```python
from build123d import *

# Parameters (mm, degrees)
F_01_RAIL_BASE_PROFILE_W   = 340
F_01_RAIL_BASE_PROFILE_H   = 130
F_01_RAIL_BASE_PROFILE_R   = 4.5
F_01_RAIL_BASE_PROFILE_W_2 = 281
F_01_RAIL_BASE_PROFILE_H_2 = 62
F_01_RAIL_BASE_DEPTH       = 10
F_02_GUIDE_RAIL_PROFILES_W = 326.4
F_02_GUIDE_RAIL_PROFILES_H = 10
F_02_GUIDE_RAILS_DEPTH     = 42


with BuildPart() as part:
    # 01_Rail_Base_Profile → 01_Rail_Base (new body)
    with BuildSketch(Plane(origin=(0, 0, 0), x_dir=(1, 0, 0), z_dir=(0, 1, 0))):
        Rectangle(F_01_RAIL_BASE_PROFILE_W, F_01_RAIL_BASE_PROFILE_H)
        with Locations(Location((-145, -52, 0), (0, 0, 270))):
            Circle(F_01_RAIL_BASE_PROFILE_R, mode=Mode.SUBTRACT)
        with Locations(Location((-145, 52, 0), (0, 0, 270))):
            Circle(F_01_RAIL_BASE_PROFILE_R, mode=Mode.SUBTRACT)
        with Locations(Location((145, -52, 0), (0, 0, 270))):
            Circle(F_01_RAIL_BASE_PROFILE_R, mode=Mode.SUBTRACT)
        with Locations(Location((145, 52, 0), (0, 0, 270))):
            Circle(F_01_RAIL_BASE_PROFILE_R, mode=Mode.SUBTRACT)
        Rectangle(F_01_RAIL_BASE_PROFILE_W_2, F_01_RAIL_BASE_PROFILE_H_2, mode=Mode.SUBTRACT)
    extrude(amount=F_01_RAIL_BASE_DEPTH)

    # 02_Guide_Rail_Profiles → 02_Guide_Rails (add)
    with BuildSketch(Plane(origin=(0, 0, 0), x_dir=(1, 0, 0), z_dir=(0, 1, 0))):
        with Locations((0, 52)):
            Rectangle(F_02_GUIDE_RAIL_PROFILES_W, F_02_GUIDE_RAIL_PROFILES_H)
        with Locations((0, -52)):
            Rectangle(F_02_GUIDE_RAIL_PROFILES_W, F_02_GUIDE_RAIL_PROFILES_H)
    extrude(amount=F_02_GUIDE_RAILS_DEPTH)


solid = part.part
```
Verification items for the finished model (mm, model axes). A direction names the side the tool comes from. Coordinates: 2 decimals unless noted, no trailing zeros. Write each loop counter-clockwise with the first axis right and the second up, starting at its lowest first coordinate (ties: lowest second). Pieces come first, ordered by that corner, then holes. Notation, with made-up numbers: M 51.5,65.25 L 67.5,65.25 A21 cw 67.5,85.25 Z; hole C 69,27.5 d11. An arc over 180 degrees is marked long. One line per item, written item: value.
Item 1: Scan lines: line 1 along Z through (x, y) = (-156, 27); line 2 along Z through (x, y) = (71.5, 3); line 3 along Y through (x, z) = (25, -46.5). Record each from-to range of solid material in increasing order.
Check sheet entries:
line 1: z = -57 to -47, 47 to 57
line 2: z = -65 to -31, 31 to 65
line 3: y = 0 to 10
Item 2: Section check B-B, the plane z = -10. Record the boundary of the cut face in (x, y), plus the area to 3 significant figures.
Check sheet entries:
outline: M -170,0 L -140.5,0 L -140.5,10 L -170,10 Z; M 140.5,0 L 170,0 L 170,10 L 140.5,10 Z
area: 590 mm^2
Item 3: Mould release check, pull along Z, two halves, no side actions. Record for faces 4 (the flat face through (-2, 5, -65)), 5 (the flat face through (-2, 5, 65)), 6 (the flat face through (-2, 26, -47)): pulls with the +Z half, pulls with the -Z half, needs draft (parallel to the pull), parting line crosses it, or undercut.
Check sheet entries:
face 4: pulls with the -Z half
face 5: pulls with the +Z half
face 6: undercut
Item 4: Section check A-A, the plane y = 22. Record the boundary of the cut face in (x, z), plus the area to 3 significant figures.
Check sheet entries:
outline: M -163.2,-57 L 163.2,-57 L 163.2,-47 L -163.2,-47 Z; M -163.2,47 L 163.2,47 L 163.2,57 L -163.2,57 Z
area: 6,530 mm^2
Item 5: Gauge pin test, flat ends, axial feed: pin 1 Ø2 at (x, y) = (27.5, 19) entering from -Z; pin 2 Ø5 at (y, z) = (25.5, -51.5) entering from -X; pin 3 Ø11 at (y, z) = (19.5, 53.5) entering from +X; pin 4 Ø4 at (x, z) = (58.5, 30) entering from -Y. Record the tip position at first contact, or that the pin passes through.
Check sheet entries:
pin 1: stops at z = -57
pin 2: stops at x = -163.2
pin 3: stops at x = 163.2
pin 4: stops at y = 0
Item 6: Access from +Z, -Z, +X, -X, +Y, -Y to the whole of each face (thin tool, end or side, straight path). Record for faces 1 (the flat face through (163.2, 26, 52)), 2 (the flat face through (-2, 26, 57)), 3 (the flat face through (-2, 26, 47)).
Check sheet entries:
face 1: +Z, -Z, +X, +Y
face 2: +Z, +X, -X, +Y
face 3: +X, -X, +Y
Item 7: Section check C-C, the plane x = -80. Record the boundary of the cut face in (y, z), plus the area to 3 significant figures.
Check sheet entries:
outline: M 0,-65 L 10,-65 L 10,-57 L 42,-57 L 42,-47 L 10,-47 L 10,-31 L 0,-31 Z; M 0,31 L 10,31 L 10,47 L 42,47 L 42,57 L 10,57 L 10,65 L 0,65 Z
area: 1,320 mm^2
Item 8: Section check D-D, the plane z = 34. Record the boundary of the cut face in (x, y), plus the area to 3 significant figures.
Check sheet entries:
outline: M -170,0 L 170,0 L 170,10 L -170,10 Z
area: 3,400 mm^2
